Input: part model. Units: mm. Frame: model coordinates. A direction names the side the tool comes from. Give positions to 0.01 mm unless a question says otherwise; leave off trailing zeros. Loops run counter-clockwise (first coordinate to the right, second up) from the corner with the lowest first, then second, coordinate; pieces in that order, holes last. Notation, with made-up numbers: (4.25, -1.75) - (35.25, -1.75) arc R17 cw to (35.25, 31.25) - close; hole circle Ø1 at (4.5, 71.5). An arc over 180 degrees is marked (long way). Answer as a JSON object with one key per item and string values.
from build123d import *

# Parameters (mm, degrees)
SKETCH1_W           = 8
SKETCH1_H           = 10.35
BOSS_EXTRUDE1_DEPTH = 6
SKETCH2_W           = 8
SKETCH2_H           = 14
BOSS_EXTRUDE2_DEPTH = 11.76
SKETCH3_W           = 1.55
SKETCH3_H           = 4.15
CUT_EXTRUDE1_DEPTH  = 6
CUT_EXTRUDE2_DEPTH  = 2
CHAMFER1_SIZE       = 2
CHAMFER1_SIZE2      = 5.494954839
FILLET1_R           = 2
FILLET2_R           = 2
FILLET3_R           = 1
FILLET5_R           = 0.5


with BuildPart() as part:
    # Sketch1 → Boss-Extrude1 (new body)
    with BuildSketch(Plane.XY):
        with Locations((4, 5.175)):
            Rectangle(SKETCH1_W, SKETCH1_H)
    extrude(amount=BOSS_EXTRUDE1_DEPTH)

    # Sketch2 → Boss-Extrude2 (add)
    with BuildSketch(Plane.XY.offset(6)):
        with Locations((4, 5.175)):
            Rectangle(SKETCH2_W, SKETCH2_H)
    extrude(amount=BOSS_EXTRUDE2_DEPTH)

    # Sketch3 → Cut-Extrude1 (cut)
    with BuildSketch(Plane(origin=(8, 0, 0), x_dir=(0, 0, -1), z_dir=(1, 0, 0))):
        with Locations((-14.985, 3.75)):
            Rectangle(SKETCH3_W, SKETCH3_H)
    extrude(amount=-CUT_EXTRUDE1_DEPTH, mode=Mode.SUBTRACT)

    # Sketch4 → Cut-Extrude2 (cut)
    with BuildSketch(Plane(origin=(8, 0, 0), x_dir=(0, 0, -1), z_dir=(1, 0, 0))):
        Polygon((-14.21, 1.675), (-11.21, 1.675), (-11.21, -1.825), (-9.21, -1.825), (-9.21, 5.825), (-14.21, 5.825), align=None)
    extrude(amount=-CUT_EXTRUDE2_DEPTH, mode=Mode.SUBTRACT)

    # Chamfer1
    chamfer1_edges = [part.edges().sort_by_distance(p)[0] for p in [
        (4, -1.825, 17.76),
        (4, 12.175, 17.76),
    ]]
    chamfer1_side = [part.faces().sort_by_distance(p)[0] for p in [
        (4, 5.175, 17.76),
    ]]
    chamfer(chamfer1_edges, length=CHAMFER1_SIZE, length2=CHAMFER1_SIZE2, reference=chamfer1_side[0])

    # Fillet1
    fillet1_edges = [part.edges().sort_by_distance(p)[0] for p in [
        (4, 0.175, 17.76),
        (4, 10.175, 17.76),
    ]]
    fillet(fillet1_edges, radius=FILLET1_R)

    # Fillet2
    fillet2_edges = [part.edges().sort_by_distance(p)[0] for p in [
        (7, 5.825, 9.21),
        (7, 1.675, 11.21),
    ]]
    fillet(fillet2_edges, radius=FILLET2_R)

    # Fillet3
    fillet3_edges = [part.edges().sort_by_distance(p)[0] for p in [
        (6, 3.75, 14.21),
    ]]
    fillet(fillet3_edges, radius=FILLET3_R)

    # Fillet5
    fillet5_edges = [part.edges().sort_by_distance(p)[0] for p in [
        (8, 10.35, 3),
        (8, 0, 3),
    ]]
    fillet(fillet5_edges, radius=FILLET5_R)


solid = part.part
Item 1: Cut plane C-C (y = 2.25). Return loops of the section in (x, z), then the cut area to 3 significant figures.
Geometry check:
{"outline": "(0, 0) - (8, 0) - (8, 9.21) - (6, 9.21) - (6, 13.21) arc R1 ccw to (5, 14.21) - (2, 14.21) - (2, 15.76) - (8, 15.76) - (8, 17.76) - (0, 17.76) - close", "area": "123 mm2"}
Item 2: Access query for faces 1 (the face through (7, 1, 9.21)), 2 (the face through (2, 4, 15)), 3 (the face through (4, 5, 17.76)). Directions: +Z, -Z, +X, -X, +Y, -Y. A direction counts if a zero-diameter tool reaches every point of the face in a straight line with its end or side. Return the directions, or none.
Geometry check:
{"face 1": "+X, -Y", "face 2": "+X", "face 3": "+Z, +X, -X, +Y, -Y"}
Item 3: Contact query for flat-ended pins moving along their axis: P1, Ø2, axis at x = 7, y = 1, coming from the +Z side; P2, Ø1.8, axis at x = 4, z = 1.5, coming from the -Y side; P3, Ø1.4, axis at x = 5.5, z = 13.5, coming from the -Y side; P4, Ø2, axis at x = 5, z = 14.5, coming from the +Y side. Output: stop coordinate, or through.
Geometry check:
{"P1": "stops at z = 17.76", "P2": "stops at y = 0", "P3": "stops at y = -1.63", "P4": "stops at y = 11.73"}
Item 4: Mould query, pull axis Z, two halves, no side actions, for faces 4 (the face through (4, -1, 6)), 5 (the face through (4, 0, 3)), 6 (the face through (6.986, 5.224, 9.78)). Classes: released by +Z, released by -Z, zero draft, split by the parting line, or undercut.
Geometry check:
{"face 4": "released by -Z", "face 5": "zero draft", "face 6": "undercut"}
Item 5: Cut plane A-A (x = 3.5). Return loops of the section in (y, z) (3 decimals).
Geometry check:
{"outline": "(-1.825, 6) - (0, 6) - (0, 0) - (10.35, 0) - (10.35, 6) - (12.175, 6) - (12.175, 12.265) - (10.654, 16.444) arc R2 ccw to (8.775, 17.76) - (1.575, 17.76) arc R2 ccw to (-0.304, 16.444) - (-1.825, 12.265) - close; hole (1.675, 14.21) - (5.825, 14.21) - (5.825, 15.76) - (1.675, 15.76) - close"}
Item 6: Material intervals for line 1 (Y direction, x = 4.25, z = 2.75); line 2 (X direction, y = 5.25, z = 10.5); line 3 (X direction, y = 1.75, z = 14.5), sorted ascending. Write a range as [from, to].
Geometry check:
{"line 1": "y = [0, 10.35]", "line 2": "x = [0, 6]", "line 3": "x = [0, 2]"}
Item 7: Cut plane D-D (x = 0.5). Return loops of the section in (y, z) (3 decimals), then the cut area to 3 significant figures.
Geometry check:
{"outline": "(-1.825, 6) - (0, 6) - (0, 0) - (10.35, 0) - (10.35, 6) - (12.175, 6) - (12.175, 12.265) - (10.654, 16.444) arc R2 ccw to (8.775, 17.76) - (1.575, 17.76) arc R2 ccw to (-0.304, 16.444) - (-1.825, 12.265) - close", "area": "215 mm2"}
Item 8: Cut plane B-B (z = 4.75). Return loops of the section in (x, y).
Geometry check:
{"outline": "(0, 0) - (7.5, 0) arc R0.5 ccw to (8, 0.5) - (8, 9.85) arc R0.5 ccw to (7.5, 10.35) - (0, 10.35) - close"}
